Can you work these out from the model? Positions are in its coordinate system, mm. Face numbers are marked on the shaded views. A direction names the side the tool comes from. Give positions to 0.01 mm unless a question says otherwise; leave off trailing zeros. Loops run counter-clockwise (first coordinate to the right, second up) from the corner with the lowest first, then second, coordinate; pieces in that order, holes last. Notation, with made-up numbers: (70, 74) - (85, 74) arc R29 cw to (85, 106) - close; hole circle Ø7 at (-10.5, 72). An arc over 180 degrees is marked (long way). Answer as a JSON object with one key per item and string values. Group by question number.
Item 1: Suppose I cut it at A-A on x = 0. Write out the boundary of the cut face in (y, z) (3 decimals).
Item 2: Please list where these lines run through material, in increasing order: L1, parallel to Y at x = 0, z = 1.15 (3 decimals); L2, parallel to Z at x = -3.25, y = -4.25; L3, parallel to Y at x = -1.5, z = 10.75.
Item 3: Suppose I cut it at D-D on y = -8.5. Write out the boundary of the cut face in (x, z).
Item 4: Suppose I cut it at C-C on x = 8. Write out the boundary of the cut face in (y, z) (3 decimals), and give its area (3 significant figures).
Item 5: Thinking about a two-plate mould opening in X: for the marked faces 5, 6 and 7, which applies, pulls with the +X half, pulls with the -X half, needs draft (parallel to the pull), parting line crosses it, or undercut?
Item 6: Suppose I cut it at B-B on y = 0. Write out the boundary of the cut face in (x, z) (3 decimals).
Item 7: Which directions (+Z, -Z, +X, -X, +Y, -Y) give clear straight access to the entire face, cutting with the end or side of a thin tool? Please do the marked faces 1, 2, 3 and 4.
Item 8: Will these pins go through, and if not, where does the flat tip stop? pin 1 (7 mm diameter, centred on x = 0, y = 0, fed in from -Z); pin 2 (10 mm diameter, centred on x = -5, z = 17, fed in from -Y); pin 3 (8 mm diameter, centred on x = -2.5, z = 19.5, fed in from +Y).
from build123d import *

# Parameters (mm, degrees)
SKETCH1_R           = 11
SKETCH1_R_2         = 1.025
SKETCH1_R_3         = 4.25
BOSS_EXTRUDE1_DEPTH = 3
SKETCH2_R           = 5
SKETCH2_R_2         = 2.5
BOSS_EXTRUDE2_DEPTH = 22
CUT_EXTRUDE1_START  = -10
CUT_EXTRUDE1_DEPTH  = 10


with BuildPart() as part:
    # Sketch1 → Boss-Extrude1 (new body)
    with BuildSketch(Plane(origin=(0, 0, 0), x_dir=(0, 1, 0), z_dir=(0, 0, 1))):
        with Locations(Location((0, 0, 0), (0, 0, 270))):
            Circle(SKETCH1_R)
        with Locations(Location((0, 8, 0), (0, 0, 270))):
            Circle(SKETCH1_R_2, mode=Mode.SUBTRACT)
        with Locations(Location((0, 0, 0), (0, 0, 270))):
            Circle(SKETCH1_R_3, mode=Mode.SUBTRACT)
        with Locations(Location((8, 0, 0), (0, 0, 270))):
            Circle(SKETCH1_R_2, mode=Mode.SUBTRACT)
        with Locations(Location((0, -8, 0), (0, 0, 270))):
            Circle(SKETCH1_R_2, mode=Mode.SUBTRACT)
        with Locations(Location((-8, 0, 0), (0, 0, 270))):
            Circle(SKETCH1_R_2, mode=Mode.SUBTRACT)
    extrude(amount=BOSS_EXTRUDE1_DEPTH)

    # Sketch2 → Boss-Extrude2 (add)
    with BuildSketch(Plane.XY.offset(3)):
        with Locations(Location((0, 0, 0), (0, 0, 180))):
            Circle(SKETCH2_R)
        with Locations(Location((0, 0, 0), (0, 0, 180))):
            Circle(SKETCH2_R_2, mode=Mode.SUBTRACT)
    extrude(amount=BOSS_EXTRUDE2_DEPTH)

    # Sketch3 → Cut-Extrude1 (cut)
    with BuildSketch(Plane.XY.offset(25).offset(CUT_EXTRUDE1_START)):
        with BuildLine():
            Line((3.5, -3.570714214), (-3.5, -3.570714214))
            ThreePointArc((-3.5, -3.570714214), (0, -5), (3.5, -3.570714214))
        make_face()
    extrude(amount=CUT_EXTRUDE1_DEPTH, mode=Mode.SUBTRACT)


solid = part.part
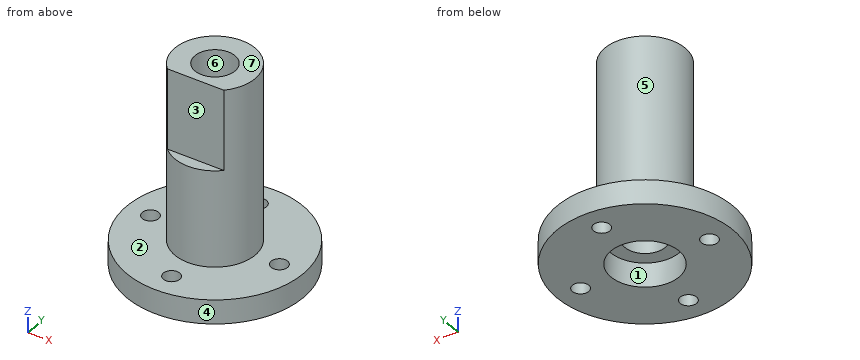
Worked out:
{
 "1": {"outline": "(-11, 0) - (-9.025, 0) - (-9.025, 3) - (-11, 3) - close; (-6.975, 0) - (-4.25, 0) - (-4.25, 3) - (-2.5, 3) - (-2.5, 25) - (-3.571, 25) - (-3.571, 15) - (-5, 15) - (-5, 3) - (-6.975, 3) - close; (2.5, 3) - (4.25, 3) - (4.25, 0) - (6.975, 0) - (6.975, 3) - (5, 3) - (5, 25) - (2.5, 25) - close; (9.025, 0) - (11, 0) - (11, 3) - (9.025, 3) - close"},
 "2": {"L1": "y = -11 to -9.025, -6.975 to -4.25, 4.25 to 6.975, 9.025 to 11", "L2": "z = 0 to 3", "L3": "y = -4.77 to -2, 2 to 4.77"},
 "3": {"outline": "(-6.98, 0) - (-0.89, 0) - (-0.89, 3) - (-6.98, 3) - close; (0.89, 0) - (6.98, 0) - (6.98, 3) - (0.89, 3) - close"},
 "4": {"outline": "(-7.55, 0) - (-1.025, 0) - (-1.025, 3) - (-7.55, 3) - close; (1.025, 0) - (7.55, 0) - (7.55, 3) - (1.025, 3) - close", "area": "39.1 mm2"},
 "5": {"face 5": "parting line crosses it", "face 6": "undercut", "face 7": "needs draft"},
 "6": {"outline": "(-11, 0) - (-9.025, 0) - (-9.025, 3) - (-11, 3) - close; (-6.975, 0) - (-4.25, 0) - (-4.25, 3) - (-2.5, 3) - (-2.5, 25) - (-5, 25) - (-5, 3) - (-6.975, 3) - close; (2.5, 3) - (4.25, 3) - (4.25, 0) - (6.975, 0) - (6.975, 3) - (5, 3) - (5, 25) - (2.5, 25) - close; (9.025, 0) - (11, 0) - (11, 3) - (9.025, 3) - close"},
 "7": {"face 1": "-Z", "face 2": "+Z", "face 3": "+Z, +X, -X, -Y", "face 4": "+Z, -Z"},
 "8": {"pin 1": "stops at z = 3", "pin 2": "stops at y = -4.98", "pin 3": "stops at y = 5"}
}
